from build123d import *

# Parameters (mm, degrees)
SKETCH1_R           = 3.375
SKETCH1_RX          = 7.5
SKETCH1_RY          = 5.3
SKETCH1_W           = 2.76
SKETCH1_H           = 1.15
BOSS_EXTRUDE1_DEPTH = 3


with BuildPart() as part:
    # Sketch1 → Boss-Extrude1 (new body)
    with BuildSketch(Plane(origin=(0, 0, 0), x_dir=(1, 0, 0), z_dir=(0, 1, 0))):
        with BuildLine():
            Line((0, 0), (35.332576055, 0))
            Line((35.332576055, 0), (35.332576055, -35))
            Line((35.332576055, -35), (0, -35))
            ThreePointArc((0, -35), (-19.284551552, -17.5), (0, 0))
        make_face()
        with Locations(Location((20.332576055, -17.5, 0), (0, 0, 270))):
            Circle(SKETCH1_R, mode=Mode.SUBTRACT)
        with Locations(Location((-4.667423945, -17.5), (0, 0, 118.629649839))):
            Ellipse(SKETCH1_RX, SKETCH1_RY, mode=Mode.SUBTRACT)
        with Locations((20.332576055, -25.378095587)):
            Rectangle(SKETCH1_W, SKETCH1_H, mode=Mode.SUBTRACT)
    extrude(amount=BOSS_EXTRUDE1_DEPTH)


solid = part.part
CAD build for the part. Positions are in the model's coordinates, mm. A direction names the side the tool comes from. Coordinates: 2 decimals unless noted, no trailing zeros. Write each loop counter-clockwise with the first axis right and the second up, starting at its lowest first coordinate (ties: lowest second). Pieces come first, ordered by that corner, then holes. Notation, with made-up numbers: M 60.5,73.25 L 84.5,73.25 A34 cw 84.5,111.25 Z; hole C 84.25,-39.75 d5. An arc over 180 degrees is marked long. Answer as a JSON object with one key per item and string values. Group by question number.
1) Saw through at C-C (z = 33). Write the cut outline in (x, y).
2) Pin check, flat tips, straight feed: pin 1 Ø1.5 at (x, y) = (11, 1.5) entering from +Z; pin 2 Ø1.5 at (x, y) = (-5.5, 1.5) entering from -Z; pin 3 Ø0.8 at (x, y) = (20.5, 1.5) entering from -Z; pin 4 Ø3 at (x, z) = (-6, 21.5) entering from +Y (3 decimals). Stop position of each tip, or through.
3) Wall check: line 1 (X direction, y = 1.25, z = 17.5); line 2 (X direction, y = 2.3, z = 15); line 3 (Z direction, x = 13, y = 2.05). Give the ranges that are in metal, low to high. Write a range as from..to.
4) Mould opens along X. For faces 1 (the face through (17, 1, 0)), 2 (the face through (20, 1, 24.803)), 3 (the face through (35.333, 1, 17)) say: +X half, -X half, draft (parallel to the pull), parting line (faces both ways), or undercut.
5) Saw through at A-A (y = 2.35). Give the number of separate pieces and of enclosed holes in the cut face, plus the area to 3 significant figures.
6) Tool access for faces 4 (the face through (8, 3, 17)), 5 (the face through (18, 1, 35)), 6 (the face through (21.713, 1, 25)): list every direction of +Z, -Z, +X, -X, +Y, -Y with a clear straight run to the whole face (end or side of a thin tool).
Values follow:
{
 "1": {"outline": "M -10,0 L 35.33,0 L 35.33,3 L -10,3 Z"},
 "2": {"pin 1": "stops at z = 35", "pin 2": "stops at z = 0.18", "pin 3": "stops at z = 0", "pin 4": "passes through"},
 "3": {"line 1": "x = -19.28..-10.3, 0.97..16.96, 23.71..35.33", "line 2": "x = -19.11..-10.53, 0.01..18.07, 22.6..35.33", "line 3": "z = 0..35"},
 "4": {"face 1": "draft", "face 2": "undercut", "face 3": "+X half"},
 "5": {"separate pieces": "1", "enclosed holes": "3", "area": "1,620 mm2"},
 "6": {"face 4": "+Z, -Z, +X, -X, +Y", "face 5": "+Z, +X, +Y, -Y", "face 6": "+Y, -Y"}
}
